```python
from build123d import *

# Parameters (mm, degrees)
BOSS_EXTRUDE1_DEPTH      = 5
BOSS_EXTRUDE1_DEPTH_BACK = 5
SKETCH1_W                = 250
SKETCH1_H                = 10
SKETCH1_H_2              = 100
SKETCH1_3_W              = 250
SKETCH1_3_H              = 100
CUT_EXTRUDE1_DEPTH       = 260.663243452
SKETCH1_4_W              = 250
SKETCH1_4_H              = 10
CUT_EXTRUDE2_DEPTH       = 2


with BuildPart() as part:
    # Sketch1 → Boss-Extrude1 (new, two sides: drawn at the far end of the back side and taken through both)
    with BuildSketch(Plane.XY.offset(-BOSS_EXTRUDE1_DEPTH_BACK)):
        with Locations((125, 55)):
            Rectangle(SKETCH1_W, SKETCH1_H)
        with Locations((125, 65)):
            Rectangle(SKETCH1_W, SKETCH1_H)
        with Locations((125, -55)):
            Rectangle(SKETCH1_W, SKETCH1_H)
        with Locations((125, -65)):
            Rectangle(SKETCH1_W, SKETCH1_H)
        with Locations((125, 0)):
            Rectangle(SKETCH1_W, SKETCH1_H_2)
    extrude(amount=BOSS_EXTRUDE1_DEPTH + BOSS_EXTRUDE1_DEPTH_BACK)

    # Sketch1_3 → Cut-Extrude1 (cut, through all)
    with BuildSketch(Plane.XY):
        with Locations((125, 0)):
            Rectangle(SKETCH1_3_W, SKETCH1_3_H)
    extrude(amount=CUT_EXTRUDE1_DEPTH, mode=Mode.SUBTRACT)

    # Sketch1_4 → Cut-Extrude2 (cut)
    with BuildSketch(Plane.XY):
        with Locations((125, 55)):
            Rectangle(SKETCH1_4_W, SKETCH1_4_H)
        with Locations((125, -55)):
            Rectangle(SKETCH1_4_W, SKETCH1_4_H)
    extrude(amount=CUT_EXTRUDE2_DEPTH, mode=Mode.SUBTRACT)


solid = part.part
```
Geometry check sheet. Reference: the model listing, model coordinates, mm. A direction names the side the tool comes from. Give positions to 0.01 mm unless a question says otherwise; leave off trailing zeros. Write each loop counter-clockwise with the first axis right and the second up, starting at its lowest first coordinate (ties: lowest second). Pieces come first, ordered by that corner, then holes. Notation, with made-up numbers: (22.25, -34) - (56.25, -34) arc R12 ccw to (56.25, -23) - close; hole circle Ø9 at (40.25, 9.5). An arc over 180 degrees is marked (long way). Use a Markdown table: item, result.
Q1. Draft check along Z on faces 3 (the face through (250, -1, -1)), 4 (the face through (123, -60, 5)), 5 (the face through (123, -55, 2)). Enter one of: pulls with the +Z half, pulls with the -Z half, needs draft (parallel to the pull), parting line crosses it, or undercut.
Computed:
| item | result |
|---|---|
| face 3 | needs draft |
| face 4 | pulls with the +Z half |
| face 5 | undercut |
Q2. Section check A-A, the plane y = -53.5. Enter the section's corners in (x, z).
Computed:
| item | result |
|---|---|
| outline | (0, -5) - (250, -5) - (250, 0) - (0, 0) - close; (0, 2) - (250, 2) - (250, 5) - (0, 5) - close |
Q3. Section check B-B, the plane x = 64. Enter the section's corners in (y, z).
Computed:
| item | result |
|---|---|
| outline | (-70, -5) - (70, -5) - (70, 5) - (50, 5) - (50, 2) - (60, 2) - (60, 0) - (-60, 0) - (-60, 2) - (-50, 2) - (-50, 5) - (-70, 5) - close |
Q4. Section check C-C, the plane y = 14. Enter the section's corners in (x, z), then the cut area to 3 significant figures.
Computed:
| item | result |
|---|---|
| outline | (0, -5) - (250, -5) - (250, 0) - (0, 0) - close |
| area | 1,250 mm² |
Q5. Go/stop test with a flat-tipped pin: P1, Ø2, axis at x = 120, y = -19.5, coming from the +Z side. Record where the tip stops, or that it passes through.
Computed:
| item | result |
|---|---|
| P1 | stops at z = 0 |
Q6. Set-up check for faces 1 (the face through (123, 1, 0)), 2 (the face through (123, -70, 0)): record each of +Z, -Z, +X, -X, +Y, -Y from which the full face is reachable in a straight line by a thin tool's end or side.
Computed:
| item | result |
|---|---|
| face 1 | +X, -X |
| face 2 | +Z, -Z, +X, -X, -Y |
Q7. Thickness scan on L1, parallel to Y at x = 132, z = 3.25; L2, parallel to Y at x = 219.5, z = 1; L3, parallel to Z at x = 69.5, y = -16. Record the ranges inside material, lowest first. Write a range as [from, to].
Computed:
| item | result |
|---|---|
| L1 | y = [-70, -50], [50, 70] |
| L2 | y = [-70, -60], [60, 70] |
| L3 | z = [-5, 0] |
